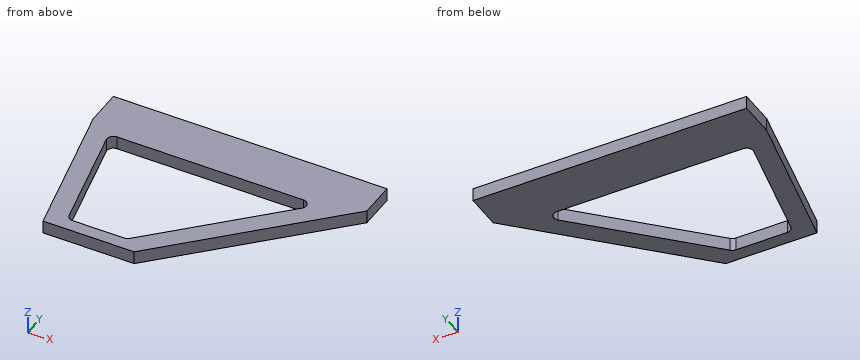
from build123d import *

# Parameters (mm, degrees)
BOSS_EXTRU_1_DEPTH = 5
FILLET1_R          = 5


with BuildPart() as part:
    # Esquisse2 → Boss.-Extru.1 (new, symmetric)
    with BuildSketch(Plane.XY):
        Polygon((-30.197209457, -50.23903484), (-5.197209457, -165.23903484), (64.802790543, -165.23903484), (179.802790543, -50.23903484), (179.802790543, -22.33903484), (-30.197209457, -22.33903484), align=None)
        Polygon((53.589587107, -155.23903484), (148.589587107, -60.23903484), (-12.672945593, -60.23903484), (7.97922832, -155.23903484), align=None, mode=Mode.SUBTRACT)
    extrude(amount=BOSS_EXTRU_1_DEPTH, both=True)

    # Fillet1
    fillet1_edges = [part.edges().sort_by_distance(p)[0] for p in [
        (7.97922832, -155.23903484, 0),
        (53.589587107, -155.23903484, 0),
        (148.589587107, -60.23903484, 0),
        (-12.672945593, -60.23903484, 0),
    ]]
    fillet(fillet1_edges, radius=FILLET1_R)


solid = part.part
Verification items for the finished model (mm, model axes). Coordinates: 2 decimals unless noted, no trailing zeros. Order: outer loops, then holes, each group sorted by start corner. A loop starts at its lowest first (then second) coordinate and runs counter-clockwise, first axis right, second up. Notation, with made-up numbers: (7, 31.25) -> (54, 31.25) arc R30 ccw to (54, 55.25) -> close; hole circle Ø4 at (55.25, 73). An arc over 180 degrees is marked (long way). Use CSV: the item, a comma, the result in double quotes. Start each with the question number.
Q1. Depth check by flat-ended pin: P1, Ø2, axis at y = -77.5, z = -0.5, coming from the -X side; P2, Ø3, axis at x = 110, z = -1, coming from the -Y side. Enter the tip coordinate at first touch or a pass-through.
Q2. Section check A-A, the plane x = 33.5. Record the cut outline in (y, z), and give its area (3 significant figures).
Q3. Section check C-C, the plane y = -116. Record the cut outline in (x, z), and give its area (3 significant figures).
Q4. Thickness scan on line 1 along Y through (x, z) = (22, -1.25); line 2 along Y through (x, z) = (61, -2.5); line 3 along X through (y, z) = (-126.5, 2.25). Record the ranges inside material, lowest first.
Q5. Section check B-B, the plane z = -0.75. Record the cut outline in (x, y).
Returned:
1,P1,"stops at x = -24.49"
1,P2,"stops at y = -121.54"
2,outline,"(-165.24, -5) -> (-155.24, -5) -> (-155.24, 5) -> (-165.24, 5) -> close; (-60.24, -5) -> (-22.34, -5) -> (-22.34, 5) -> (-60.24, 5) -> close"
2,area,"479 mm^2"
3,outline,"(-15.9, -5) -> (-0.55, -5) -> (-0.55, 5) -> (-15.9, 5) -> close; (92.83, -5) -> (114.04, -5) -> (114.04, 5) -> (92.83, 5) -> close"
3,area,"366 mm^2"
4,line 1,"y = -165.24 to -155.24, -60.24 to -22.34"
4,line 2,"y = -165.24 to -147.83, -60.24 to -22.34"
4,line 3,"x = -13.62 to 1.73, 82.33 to 103.54"
5,outline,"(-30.2, -50.24) -> (-5.2, -165.24) -> (64.8, -165.24) -> (179.8, -50.24) -> (179.8, -22.34) -> (-30.2, -22.34) -> close; hole (-11.36, -66.3) -> (7.12, -151.3) arc R5 ccw to (12.01, -155.24) -> (51.52, -155.24) arc R5 ccw to (55.05, -153.77) -> (140.05, -68.77) arc R5 ccw to (136.52, -60.24) -> (-6.47, -60.24) arc R5 ccw to start"
